The model under review builds one solid part; all positions refer to its coordinate system, in mm. Coordinates: 2 decimals unless noted, no trailing zeros. Loops run counter-clockwise (first coordinate to the right, second up) from the corner with the lowest first, then second, coordinate; pieces in that order, holes last. Notation, with made-up numbers: M -31,25 L 1,25 A9 ccw 1,40 Z; hole C 38.5,48 d8. An arc over 180 degrees is marked long. Return JSON: item names as keys, results as strings.
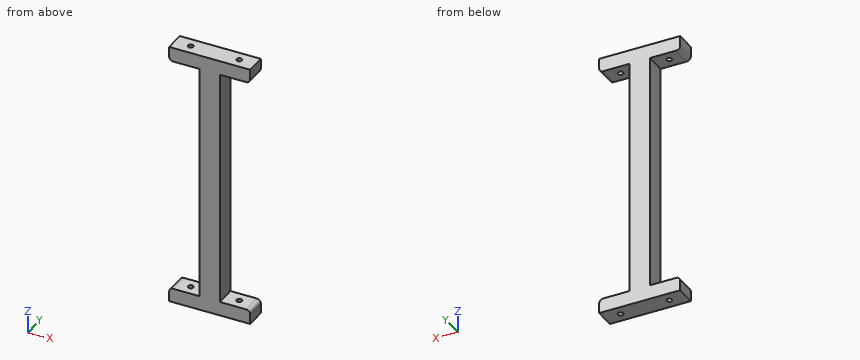
```python
from build123d import *

# Parameters (mm, degrees)
CYLINDER010_R     = 1.3
CYLINDER010_DEPTH = 146
CYLINDER008_R     = 1.3
CYLINDER008_DEPTH = 146
BOX067_W          = 15
BOX067_H          = 10
BOX067_DEPTH      = 7
BOX068_W          = 10
BOX068_H          = 10
BOX068_DEPTH      = 132
BOX070_W          = 15
BOX070_H          = 10
BOX070_DEPTH      = 7
BOX071_W          = 15
BOX071_H          = 10
BOX071_DEPTH      = 7
BOX069_W          = 15
BOX069_H          = 10
BOX069_DEPTH      = 7
FILLET001_R       = 2


with BuildPart() as cilindro010:
    # Cylinder010 → Cylinder010 (new body)
    with BuildSketch(Plane(origin=(182, 5, 8), x_dir=(1, 0, 0), z_dir=(0, 0, 1))):
        Circle(CYLINDER010_R)
    extrude(amount=CYLINDER010_DEPTH)


with BuildPart() as cilindro008:
    # Cylinder008 → Cylinder008 (new body)
    with BuildSketch(Plane(origin=(158, 5, 8), x_dir=(1, 0, 0), z_dir=(0, 0, 1))):
        Circle(CYLINDER008_R)
    extrude(amount=CYLINDER008_DEPTH)


with BuildPart() as cubo030:
    # Box067 → Box067 (new body)
    with BuildSketch(Plane(origin=(175, 0, 15), x_dir=(1, 0, 0), z_dir=(0, 0, 1))):
        with Locations((7.5, 5)):
            Rectangle(BOX067_W, BOX067_H)
    extrude(amount=BOX067_DEPTH)


with BuildPart() as cubo031:
    # Box068 → Box068 (new body)
    with BuildSketch(Plane(origin=(165, 0, 15), x_dir=(1, 0, 0), z_dir=(0, 0, 1))):
        with Locations((5, 5)):
            Rectangle(BOX068_W, BOX068_H)
    extrude(amount=BOX068_DEPTH)


with BuildPart() as cubo033:
    # Box070 → Box070 (new body)
    with BuildSketch(Plane(origin=(150, 0, 15), x_dir=(1, 0, 0), z_dir=(0, 0, 1))):
        with Locations((7.5, 5)):
            Rectangle(BOX070_W, BOX070_H)
    extrude(amount=BOX070_DEPTH)


with BuildPart() as cubo034:
    # Box071 → Box071 (new body)
    with BuildSketch(Plane(origin=(150, 0, 140), x_dir=(1, 0, 0), z_dir=(0, 0, 1))):
        with Locations((7.5, 5)):
            Rectangle(BOX071_W, BOX071_H)
    extrude(amount=BOX071_DEPTH)


with BuildPart() as obj1:
    # Box069 → Box069 (new body)
    with BuildSketch(Plane(origin=(175, 0, 140), x_dir=(1, 0, 0), z_dir=(0, 0, 1))):
        with Locations((7.5, 5)):
            Rectangle(BOX069_W, BOX069_H)
    extrude(amount=BOX069_DEPTH)

    # Fusion009: union Cubo030, Cubo031, Cubo033, Cubo034
    add(cubo030.part)
    add(cubo031.part)
    add(cubo033.part)
    add(cubo034.part)

    # Fillet001
    fillet001_edges = [obj1.edges().sort_by_distance(p)[0] for p in [
        (190, 5, 140),
        (190, 5, 22),
        (150, 5, 22),
        (150, 5, 140),
    ]]
    fillet(fillet001_edges, radius=FILLET001_R)

    # Cut022: cut Cilindro008
    add(cilindro008.part, mode=Mode.SUBTRACT)

    # Cut025: cut Cilindro010
    add(cilindro010.part, mode=Mode.SUBTRACT)


solid = obj1.part
```
1. Add section A-A on x = 179. Give the boundary of the cut face in (y, z), plus the area to 3 significant figures.
Check values:
{"outline": "M 0,15 L 10,15 L 10,22 L 0,22 Z; M 0,140 L 10,140 L 10,147 L 0,147 Z", "area": "140 mm²"}
2. Add section D-D on z = 108.5. Give the boundary of the cut face in (x, y), plus the area to 3 significant figures.
Check values:
{"outline": "M 165,0 L 175,0 L 175,10 L 165,10 Z", "area": "100 mm²"}
3. Add section C-C on x = 158. Give the boundary of the cut face in (y, z), plus the area to 3 significant figures.
Check values:
{"outline": "M 0,15 L 3.7,15 L 3.7,22 L 0,22 Z; M 0,140 L 3.7,140 L 3.7,147 L 0,147 Z; M 6.3,15 L 10,15 L 10,22 L 6.3,22 Z; M 6.3,140 L 10,140 L 10,147 L 6.3,147 Z", "area": "104 mm²"}
4. Add section B-B on y = 5. State how many separate pieces and enclosed holes the cut face has, plus the area to 3 significant figures.
Check values:
{"separate pieces": "5", "enclosed holes": "0", "area": "1,660 mm²"}
5. To check wall thickness, follow line 1 (X direction, y = 5, z = 144.75); line 2 (Z direction, x = 185, y = 8); line 3 (Y direction, x = 158, z = 18.75). State the ranges of each line that lie inside material, in increasing order.
Check values:
{"line 1": "150 to 156.7, 159.3 to 180.7, 183.3 to 190", "line 2": "15 to 22, 140 to 147", "line 3": "0 to 3.7, 6.3 to 10"}
6. Insertion check: pin 1 Ø3 at (x, y) = (182, 5) entering from +Z; pin 2 Ø5 at (y, z) = (4, 89.5) entering from +X. Each pin has a flat end and moves straight along its axis. Give the tip position at first contact, or say it passes through.
Check values:
{"pin 1": "z = 147", "pin 2": "x = 175"}
